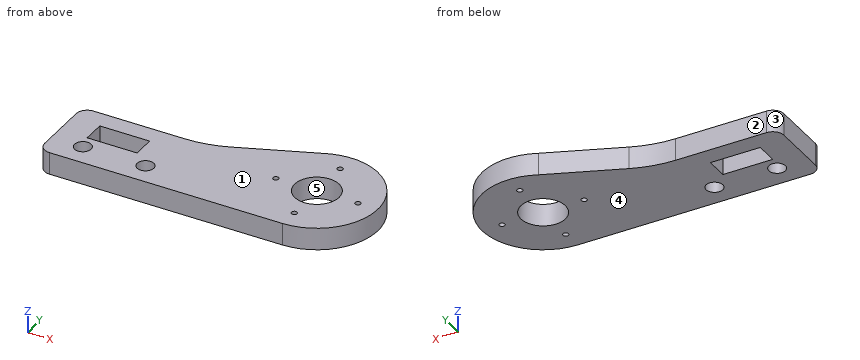
from build123d import *

# Parameters (mm, degrees)
SKETCH1_R           = 4
SKETCH1_R_2         = 0.5
SKETCH1_R_3         = 1.5
SKETCH1_W           = 9
SKETCH1_H           = 4
BOSS_EXTRUDE1_DEPTH = 4


with BuildPart() as part:
    # Sketch1 → Boss-Extrude1 (new body)
    with BuildSketch(Plane.XY):
        with BuildLine():
            Line((2, 2), (2, 12))
            ThreePointArc((2, 12), (2.585786438, 13.414213562), (4, 14))
            Line((4, 14), (20.401115249, 14))
            ThreePointArc((20.401115249, 14), (24.259789892, 14.375764219), (27.973469349, 15.488937))
            Line((27.973469349, 15.488937), (41.227821741, 20.910918962))
            ThreePointArc((41.227821741, 20.910918962), (56.724274068, 13.447436559), (46, 0))
            Line((46, 0), (4, 0))
            ThreePointArc((4, 0), (2.585786438, 0.585786438), (2, 2))
        make_face()
        with Locations((46, 11)):
            Circle(SKETCH1_R, mode=Mode.SUBTRACT)
        with Locations((46, 18.4)):
            Circle(SKETCH1_R_2, mode=Mode.SUBTRACT)
        with Locations((46.121025162, 3.600989734)):
            Circle(SKETCH1_R_2, mode=Mode.SUBTRACT)
        with Locations((53.4, 11)):
            Circle(SKETCH1_R_2, mode=Mode.SUBTRACT)
        with Locations((38.6, 11)):
            Circle(SKETCH1_R_2, mode=Mode.SUBTRACT)
        with Locations((19, 4.1)):
            Circle(SKETCH1_R_3, mode=Mode.SUBTRACT)
        with Locations((7.7, 4.1)):
            Circle(SKETCH1_R_3, mode=Mode.SUBTRACT)
        with Locations((11.5, 8.7)):
            Rectangle(SKETCH1_W, SKETCH1_H, mode=Mode.SUBTRACT)
    extrude(amount=BOSS_EXTRUDE1_DEPTH)


solid = part.part
Model file for the job. Use its own axes, mm. Face numbers are marked on the shaded views. A direction names the side the tool comes from. Coordinates: 2 decimals unless noted, no trailing zeros. Order: outer loops, then holes, each group sorted by start corner. A loop starts at its lowest first (then second) coordinate and runs counter-clockwise, first axis right, second up. Notation, with made-up numbers: M 60.25,35 L 83.25,35 A8 cw 83.25,50 Z; hole C -26.75,11 d8. An arc over 180 degrees is marked long. Return JSON: item names as keys, results as strings.
1. Saw through at B-B (y = 8.75). Give the cut face in (x, z).
Ans:
{"outline": "M 2,0 L 7,0 L 7,4 L 2,4 Z; M 16,0 L 42.69,0 L 42.69,4 L 16,4 Z; M 49.31,0 L 56.77,0 L 56.77,4 L 49.31,4 Z"}
2. Tool access for the marked faces 1 and 2: list every direction of +Z, -Z, +X, -X, +Y, -Y with a clear straight run to the whole face (end or side of a thin tool).
Ans:
{"face 1": "+Z, +X, -X, +Y, -Y", "face 2": "+Z, -Z, -X, +Y"}
3. Saw through at A-A (x = 10.5). Give the cut face in (y, z).
Ans:
{"outline": "M 0,0 L 6.7,0 L 6.7,4 L 0,4 Z; M 10.7,0 L 14,0 L 14,4 L 10.7,4 Z"}
4. Flat gauge pin, fed straight in: pin 1 (2 mm diameter, centred on x = 8.5, z = 1.5, fed in from +Y). Where does the tip first touch, or does it go through?
Ans:
{"pin 1": "y = 14"}
5. Saw through at D-D (x = 53.4). Give the cut face in (y, z), and give its area (3 significant figures).
Ans:
{"outline": "M 2.86,0 L 10.5,0 L 10.5,4 L 2.86,4 Z; M 11.5,0 L 19.14,0 L 19.14,4 L 11.5,4 Z", "area": "61.1 mm^2"}
6. Pull direction X, two halves, no side cores. Call the marked faces 3, 4 and 5: +X half, -X half, draft (parallel to the pull), parting line (faces both ways), or undercut.
Ans:
{"face 3": "-X half", "face 4": "draft", "face 5": "undercut"}
7. Saw through at C-C (z = 2.1). Give the number of separate pieces and of enclosed holes in the cut face, and give its area (3 significant figures).
Ans:
{"separate pieces": "1", "enclosed holes": "8", "area": "797 mm^2"}
8. Drill centre lines: probe 1 along Y at (x, z) = (7.7, 0.9); probe 2 along Y at (x, z) = (19, 0.8); probe 3 along Y at (x, z) = (46, 2). Where is each one in solid material? Low to high.
Ans:
{"probe 1": "0 to 2.6, 5.6 to 6.7, 10.7 to 14", "probe 2": "0 to 2.6, 5.6 to 14", "probe 3": "0 to 3.12, 4.09 to 7, 15 to 17.9, 18.9 to 22"}
